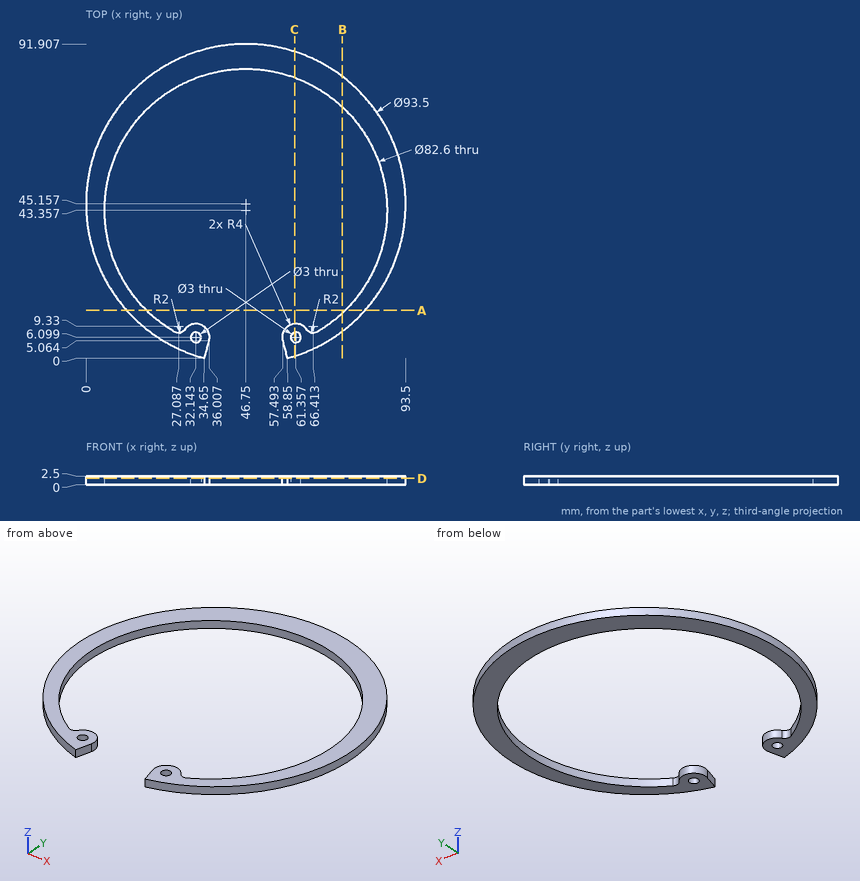
Verification items for this drawing (mm, ordinates from the low corner). Coordinates: 2 decimals unless noted, no trailing zeros. Loops run counter-clockwise (first coordinate to the right, second up) from the corner with the lowest first, then second, coordinate; pieces in that order, holes last.
Item 1: Sectioned sample at A-A, the plane y = 14. Record the boundary of the cut face in (x, z).
Item 2: Sectioned sample at D-D, the plane z = 1.9. Record the boundary of the cut face in (x, y).
Item 3: Sectioned sample at C-C, the plane x = 61. Record the boundary of the cut face in (y, z).
Item 4: Go/stop test with a flat-tipped pin: pin 1 Ø2.5 at (x, y) = (61.36, 6.1) entering from +Z. Record where the tip stops, or that it passes through.
Item 5: Sectioned sample at B-B, the plane x = 75. Record the boundary of the cut face in (y, z).
Item 6: Thickness scan on line 1 (X direction, y = 43, z = 0.2); line 2 (Y direction, x = 31, z = 1.3) (1 decimal); line 3 (Y direction, x = 14.5, z = 1.05) (1 decimal). Record the ranges inside material, lowest first.
Check result:
1. outline: (11.9, 0) - (17.7, 0) - (17.7, 2.5) - (11.9, 2.5) - close; (75.8, 0) - (81.6, 0) - (81.6, 2.5) - (75.8, 2.5) - close
2. outline: (26.09, 7.6) arc R41.3 cw (long way) to (67.41, 7.6) arc R2 cw to (64.73, 8.25) arc R4 ccw to (57.49, 5.06) - (58.85, 0) arc R46.75 ccw (long way) to (34.65, 0) - (36.01, 5.06) arc R4 ccw to (28.77, 8.25) arc R2 cw to start; hole circle Ø3 at (32.14, 6.1); hole circle Ø3 at (61.36, 6.1)
3. outline: (0.63, 0) - (4.64, 0) - (4.64, 2.5) - (0.63, 2.5) - close; (7.56, 0) - (10.08, 0) - (10.08, 2.5) - (7.56, 2.5) - close; (82.12, 0) - (89.68, 0) - (89.68, 2.5) - (82.12, 2.5) - close
4. pin 1: passes through
5. outline: (7.91, 0) - (13.23, 0) - (13.23, 2.5) - (7.91, 2.5) - close; (73.48, 0) - (82.41, 0) - (82.41, 2.5) - (73.48, 2.5) - close
6. line 1: x = 0.05 to 5.45, 88.05 to 93.45
6. line 2: y = 1.1 to 5.1, 7.1 to 9.9, 81.5 to 89.2
6. line 3: y = 11.3 to 17.6, 69.2 to 79
